Design review of the part shown in the three views and the two pictorial views. Dimensions are in mm from the part's minimum x, y and z. Coordinates: 2 decimals unless noted, no trailing zeros. Loops run counter-clockwise (first coordinate to the right, second up) from the corner with the lowest first, then second, coordinate; pieces in that order, holes last. Notation, with made-up numbers: (49.5, 21.25) -> (66.5, 21.25) arc R26 ccw to (66.5, 54.25) -> close; hole circle Ø2 at (-12, 7). An arc over 180 degrees is marked (long way). One line per item, written item: value.
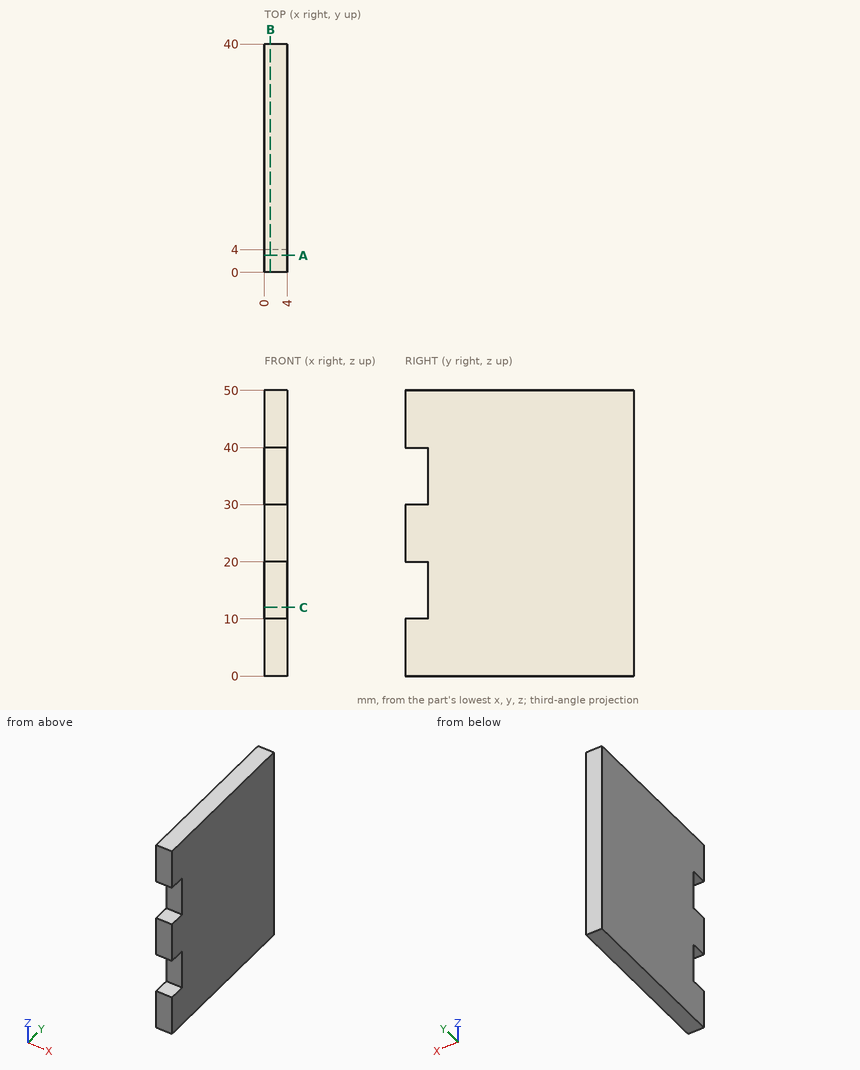
1. Take a section at B-B, the plane x = 1.05. Give the boundary of the cut face in (y, z), and give its area (3 significant figures).
Return value:
outline: (0, 0) -> (40, 0) -> (40, 50) -> (0, 50) -> (0, 40) -> (4, 40) -> (4, 30) -> (0, 30) -> (0, 20) -> (4, 20) -> (4, 10) -> (0, 10) -> close
area: 1,920 mm2
2. Take a section at A-A, the plane y = 3. Give the boundary of the cut face in (x, z).
Return value:
outline: (0, 0) -> (4, 0) -> (4, 10) -> (0, 10) -> close; (0, 20) -> (4, 20) -> (4, 30) -> (0, 30) -> close; (0, 40) -> (4, 40) -> (4, 50) -> (0, 50) -> close
3. Take a section at C-C, the plane z = 12. Give the boundary of the cut face in (x, y), and give its area (3 significant figures).
Return value:
outline: (0, 4) -> (4, 4) -> (4, 40) -> (0, 40) -> close
area: 144 mm2
4. Insertion check: pin 1 Ø2 at (x, z) = (2, 14.5) entering from -Y. The pin has a flat end and moves straight along its axis. Give the tip position at first contact, or say it passes through.
Return value:
pin 1: stops at y = 4
5. To check wall thickness, follow probe 1 along Z at (x, y) = (2.3, 2.5); probe 2 along Y at (x, z) = (1.25, 18). State the ranges of each line that lie inside material, in increasing order. Write a range as from..to.
Return value:
probe 1: z = 0..10, 20..30, 40..50
probe 2: y = 4..40
